from build123d import *

# Parameters (mm, degrees)
PAD_DEPTH    = 20
SKETCH001_R  = 2.969433
POCKET_DEPTH = 20.001


with BuildPart() as part:
    # Sketch → Pad (new body)
    with BuildSketch(Plane.XZ):
        with BuildLine():
            ThreePointArc((14.995451, 1e-06), (0, 14.630607), (-14.995451, 1e-06))
            Line((-14.995451, 1e-06), (-19.357943, 1e-06))
            Line((-19.357943, 1e-06), (-19.357943, 39.209084))
            Line((-19.357943, 39.209084), (19.357943, 39.209084))
            Line((19.357943, 39.209084), (19.357943, 1e-06))
            Line((14.995451, 1e-06), (19.357943, 1e-06))
        make_face()
    extrude(amount=PAD_DEPTH)

    # Sketch001 → Pocket (cut, through all)
    with BuildSketch(Plane.XZ.offset(20)):
        with Locations((-0.123295, 30)):
            Circle(SKETCH001_R)
    extrude(amount=-POCKET_DEPTH, mode=Mode.SUBTRACT)


solid = part.part
Verification items for the finished model (mm, model axes). Give positions to 0.01 mm unless a question says otherwise; leave off trailing zeros. Loops run counter-clockwise (first coordinate to the right, second up) from the corner with the lowest first, then second, coordinate; pieces in that order, holes last.
1) Sectioned sample at D-D, the plane x = -7.5. Enter the section's corners in (y, z), then the cut area to 3 significant figures.
2) Sectioned sample at C-C, the plane x = 0. Enter the section's corners in (y, z), then the cut area to 3 significant figures.
3) Draft check along X on faces 1 (the flat face through (17, -10, 0)), 2 (the cylindrical face through (0.325, -9.86, 14.627)), 3 (the flat face through (-19.358, -10, 19)). Enter one of: pulls with the +X half, pulls with the -X half, needs draft (parallel to the pull), parting line crosses it, or undercut.
4) Sectioned sample at A-A, the plane z = 30. Enter the section's corners in (x, y).
5) Thickness scan on line 1 along X through (y, z) = (-15.5, 2); line 2 along Z through (x, y) = (2.5, -5); line 3 along X through (y, z) = (-7.25, 31.5). Record the ranges inside material, lowest first.
6) Depth check by flat-ended pin: pin 1 Ø10 at (x, z) = (-2, 31) entering from +Y. Enter the tip coordinate at first touch or a pass-through.
Answers:
1. outline: (-20, 12.62) - (0, 12.62) - (0, 39.21) - (-20, 39.21) - close
1. area: 532 mm2
2. outline: (-20, 14.63) - (0, 14.63) - (0, 27.03) - (-20, 27.03) - close; (-20, 32.97) - (0, 32.97) - (0, 39.21) - (-20, 39.21) - close
2. area: 373 mm2
3. face 1: needs draft
3. face 2: undercut
3. face 3: pulls with the -X half
4. outline: (-19.36, -20) - (-3.09, -20) - (-3.09, 0) - (-19.36, 0) - close; (2.85, -20) - (19.36, -20) - (19.36, 0) - (2.85, 0) - close
5. line 1: x = -19.36 to -14.81, 14.81 to 19.36
5. line 2: z = 14.42 to 28.61, 31.39 to 39.21
5. line 3: x = -19.36 to -2.69, 2.44 to 19.36
6. pin 1: stops at y = 0
